```python
from build123d import *

# Parameters (mm, degrees)
F0_R      = 2.3495
F1_DEPTH  = 15.6718
F3_R      = 2.5273
F4_DEPTH  = 0.5588
F5_DEPTH  = 12.7
F6_R      = 2.9464
F7_DEPTH  = 8.5598
F8_R      = 12.7
F9_DEPTH  = 7.5184
F10_W     = 1.4605
F10_H     = 1.8034
F10_W_2   = 1.8034
F10_H_2   = 1.4605
F11_DEPTH = 7.5184
F12_R     = 0.7358522938
F13_R     = 0.6745312693
F14_R     = 1.7145
F15_DEPTH = 5.8674


with BuildPart() as f1:
    # F0 (on Top) → F1 (new body)
    with BuildSketch(Plane.XY):
        Circle(F0_R)
    extrude(amount=F1_DEPTH)

    # F3 (on face) → F4 (join)
    with BuildSketch(Plane(origin=(0, 0, 0), x_dir=(1, 0, 0), z_dir=(0, 0, -1))):
        Circle(F3_R)
    extrude(amount=-F4_DEPTH)

    # F2 (on Front) → F5 (cut, symmetric)
    with BuildSketch(Plane.XZ):
        with BuildLine():
            Line((-0.5461, -2.8702), (0.5461, -2.8702))
            Line((0.5461, -2.8702), (0.5461, 2.8702))
            ThreePointArc((0.5461, 2.8702), (0, 2.3241), (-0.5461, 2.8702))
            Line((-0.5461, 2.8702), (-0.5461, -2.8702))
        make_face()
        with BuildLine():
            ThreePointArc((-0.5461, 2.8702), (0, 2.3241), (0.5461, 2.8702))
            Line((0.5461, 2.8702), (-0.5461, 2.8702))
        make_face()
        with BuildLine():
            Line((-0.5461, 2.8702), (0.5461, 2.8702))
            ThreePointArc((0.5461, 2.8702), (0, 3.4163), (-0.5461, 2.8702))
        make_face()
    extrude(amount=F5_DEPTH, both=True, mode=Mode.SUBTRACT)

    # F6 (on face) → F7 (join)
    with BuildSketch(Plane.XY.offset(15.6718)):
        Circle(F6_R)
    extrude(amount=-F7_DEPTH)

    # F8 (on face) → F9 (cut)
    with BuildSketch(Plane.XY.offset(15.6718)):
        Circle(F8_R)
    extrude(amount=-F9_DEPTH, mode=Mode.SUBTRACT)

    # F10 (on face) → F11 (join)
    with BuildSketch(Plane.XY.offset(8.1534)):
        with Locations((1.63195, 0)):
            Rectangle(F10_W, F10_H)
        with Locations((0, -1.63195)):
            Rectangle(F10_W_2, F10_H_2)
        Rectangle(F10_W_2, F10_H)
        with Locations((-1.63195, 0)):
            Rectangle(F10_W, F10_H)
        with Locations((0, 1.63195)):
            Rectangle(F10_W_2, F10_H_2)
    extrude(amount=F11_DEPTH)

    # F12
    f12_edges = [f1.edges().sort_by_distance(p)[0] for p in [
        (-0.9017, -0.9017, 11.9126),
        (0.9017, 0.9017, 11.9126),
        (0.9017, -0.9017, 11.9126),
        (-0.9017, 0.9017, 11.9126),
    ]]
    fillet(f12_edges, radius=F12_R)

    # F13
    f13_edges = [f1.edges().sort_by_distance(p)[0] for p in [
        (1.999876, -0.9017, 15.6718),
        (1.117226, -1.117226, 15.6718),
        (2.3622, 0, 15.6718),
        (0.9017, -1.999876, 15.6718),
        (1.999876, 0.9017, 15.6718),
        (0, -2.3622, 15.6718),
        (1.117226, 1.117226, 15.6718),
        (-0.9017, -1.999876, 15.6718),
        (0.9017, 1.999876, 15.6718),
        (-1.117226, -1.117226, 15.6718),
        (0, 2.3622, 15.6718),
        (-1.999876, -0.9017, 15.6718),
        (-0.9017, 1.999876, 15.6718),
        (-2.3622, 0, 15.6718),
        (-1.117226, 1.117226, 15.6718),
        (-1.999876, 0.9017, 15.6718),
    ]]
    fillet(f13_edges, radius=F13_R)

    # F14 (on face) → F15 (cut)
    with BuildSketch(Plane(origin=(0, 0, 0), x_dir=(1, 0, 0), z_dir=(0, 0, -1))):
        Circle(F14_R)
    extrude(amount=-F15_DEPTH, mode=Mode.SUBTRACT)


solid = f1.part
```
Part model, mm, in its own coordinate system. A direction names the side the tool comes from. Give positions to 0.01 mm unless a question says otherwise; leave off trailing zeros. Write each loop counter-clockwise with the first axis right and the second up, starting at its lowest first coordinate (ties: lowest second). Pieces come first, ordered by that corner, then holes. Notation, with made-up numbers: (-11.5, 83) -> (27.5, 83) arc R23 cw to (27.5, 120) -> close; hole circle Ø1 at (-21, 15). An arc over 180 degrees is marked (long way). Put each result on its own line as item: value. Start each with the question number.
Item 1: Wall check: L1, parallel to X at y = 0, z = 3.45; L2, parallel to X at y = -0.75, z = 12.25. Give the ranges that are in metal, low to high. Write a range as [from, to].
Item 2: Cut at C-C (y = 0). List the corners of the cut face in (x, z).
Item 3: Cut at D-D (z = 6.75). List the corners of the cut face in (x, y).
Item 4: Pin check, flat tips, straight feed: pin 1 Ø0.6 at (x, z) = (-2, 11.5) entering from -Y; pin 2 Ø0.7 at (y, z) = (2, 2) entering from -X; pin 3 Ø1 at (x, z) = (-2, 7) entering from -Y. Stop position of each tip, or through.
Item 5: Pull direction X, two halves, no side cores. Call faces 4 (the face through (-0.546, 2, 1)), 5 (the face through (2, 0, 0)), 6 (the face through (0.546, 2, 1)), 7 (the face through (2.527, 0.048, 0.275)): pulls with the +X half, pulls with the -X half, needs draft (parallel to the pull), parting line crosses it, or undercut.
Item 6: Cut at A-A (x = 0). List the corners of the cut face in (y, z), then the cut area to 3 significant figures.
Item 7: Which spindle directions (+Z, -Z, +X, -X, +Y, -Y) get a long thin tool onto all of the face, cutting with end or side? Do faces 1 (the face through (1.3, -1.3, 8.153)), 2 (the face through (0, -2.362, 12)), 3 (the face through (1.635, -0.515, 2.893)). Say none if no direction does.
Item 8: Cut at B-B (z = 13.75). List the corners of the cut face in (x, y), then the cut area to 3 significant figures.
Answer list:
1. L1: x = [-2.35, -1.71], [1.71, 2.35]
1. L2: x = [-2.36, 2.36]
2. outline: (-2.95, 7.11) -> (-2.35, 7.11) -> (-2.35, 0.56) -> (-2.53, 0.56) -> (-2.53, 0) -> (-1.71, 0) -> (-1.71, 5.87) -> (1.71, 5.87) -> (1.71, 0) -> (2.53, 0) -> (2.53, 0.56) -> (2.35, 0.56) -> (2.35, 7.11) -> (2.95, 7.11) -> (2.95, 8.15) -> (2.36, 8.15) -> (2.36, 15) arc R0.67 ccw to (1.69, 15.67) -> (-1.69, 15.67) arc R0.67 ccw to (-2.36, 15) -> (-2.36, 8.15) -> (-2.95, 8.15) -> close
3. outline: circle Ø4.7 at (0, 0)
4. pin 1: stops at y = -0.9
4. pin 2: stops at x = -1.67
4. pin 3: stops at y = -2.53
5. face 4: undercut
5. face 5: needs draft
5. face 6: undercut
5. face 7: pulls with the +X half
6. outline: (-2.95, 7.11) -> (-2.35, 7.11) -> (-2.35, 3.42) -> (-1.71, 3.42) -> (-1.71, 5.87) -> (1.71, 5.87) -> (1.71, 3.42) -> (2.35, 3.42) -> (2.35, 7.11) -> (2.95, 7.11) -> (2.95, 8.15) -> (2.36, 8.15) -> (2.36, 15) arc R0.67 ccw to (1.69, 15.67) -> (-1.69, 15.67) arc R0.67 ccw to (-2.36, 15) -> (-2.36, 8.15) -> (-2.95, 8.15) -> close
6. area: 50.4 mm2
7. face 1: +Z
7. face 2: +Z, +X, -X, -Y
7. face 3: -Z
8. outline: (-2.36, -0.9) -> (-1.64, -0.9) arc R0.74 cw to (-0.9, -1.64) -> (-0.9, -2.36) -> (0.9, -2.36) -> (0.9, -1.64) arc R0.74 cw to (1.64, -0.9) -> (2.36, -0.9) -> (2.36, 0.9) -> (1.64, 0.9) arc R0.74 cw to (0.9, 1.64) -> (0.9, 2.36) -> (-0.9, 2.36) -> (-0.9, 1.64) arc R0.74 cw to (-1.64, 0.9) -> (-2.36, 0.9) -> close
8. area: 14.3 mm2
